Could you check a few things on this model? Use its own coordinates, in mm. A direction names the side the tool comes from. Give positions to 0.01 mm unless a question says otherwise; leave off trailing zeros. Write each loop counter-clockwise with the first axis right and the second up, starting at its lowest first coordinate (ties: lowest second). Pieces come first, ordered by that corner, then holes. Notation, with made-up numbers: (-17.75, 40.5) -> (-5.75, 40.5) arc R7 ccw to (-5.75, 51.5) -> close; hole circle Ø11 at (66, 79.25). An arc over 180 degrees is marked (long way). Write item = value, one per line. Start each with the question number.
```python
from build123d import *

# Parameters (mm, degrees)
SKETCH1_R               = 31.75
BOSS_EXTRUDE1_DEPTH     = 19.05
SKETCH2_R               = 31.75
SKETCH2_R_2             = 19.05
CUT_EXTRUDE_THIN1_DEPTH = 12.7
CUT_EXTRUDE1_DEPTH      = 49.775275499
CUT_EXTRUDE1_DEPTH_BACK = 49.775275499
SKETCH3_R               = 11
SKETCH6_R               = 11
SKETCH6_R_2             = 8.46
EXTRUDE_THIN1_DEPTH     = 12.05


with BuildPart() as part:
    # Sketch1 → Boss-Extrude1 (new, symmetric)
    with BuildSketch(Plane(origin=(0, 0, 0), x_dir=(1, 0, 0), z_dir=(0, 1, 0))):
        with Locations(Location((0, 0, 0), (0, 0, 90))):
            Circle(SKETCH1_R)
    extrude(amount=BOSS_EXTRUDE1_DEPTH, both=True)

    # Sketch2 → Cut-Extrude-Thin1 (cut, symmetric)
    with BuildSketch(Plane(origin=(0, 0, 0), x_dir=(1, 0, 0), z_dir=(0, 1, 0))):
        Circle(SKETCH2_R)
        Circle(SKETCH2_R_2, mode=Mode.SUBTRACT)
    extrude(amount=CUT_EXTRUDE_THIN1_DEPTH, both=True, mode=Mode.SUBTRACT)

    # Sketch3 → Cut-Extrude1 (cut, two sides: drawn at the far end of the back side and taken through both)
    with BuildSketch(Plane(origin=(0, 0, 0), x_dir=(1, 0, 0), z_dir=(0, 1, 0)).offset(-CUT_EXTRUDE1_DEPTH_BACK)):
        with Locations(Location((0, 0, 0), (0, 0, 270))):
            Circle(SKETCH3_R)
    extrude(amount=CUT_EXTRUDE1_DEPTH + CUT_EXTRUDE1_DEPTH_BACK, mode=Mode.SUBTRACT)

    # Sketch6 → Extrude-Thin1 (add, symmetric)
    with BuildSketch(Plane(origin=(0, 0, 0), x_dir=(1, 0, 0), z_dir=(0, 1, 0))):
        Circle(SKETCH6_R)
        Circle(SKETCH6_R_2, mode=Mode.SUBTRACT)
    extrude(amount=EXTRUDE_THIN1_DEPTH, both=True)


solid = part.part
```
(1) On a 3-axis mill with a long thin cutter (end or side, diameter ignored), from which of +Z, -Z, +X, -X, +Y, -Y can I reach the whole of each face in a straight line? I mean faces 5 (the flat face through (5.7, -12.05, 6.5)), 6 (the flat face through (14, 19.05, 0)), 7 (the flat face through (14, 12.7, 14)), 8 (the cylindrical face through (3.304, 15.501, 10.492)). Say none if no direction works.
(2) Imagine slicing it at D-D (x = 0). Please give me the cut outline in (y, z), then the cut area to 3 significant figures.
(3) I'm going to push flat-ended pins straight in: pin 1 (5 mm diameter, centred on x = 6, z = 3, fed in from -Y); pin 2 (19.5 mm diameter, centred on x = 0, z = 0, fed in from +Y); pin 3 (4 mm diameter, centred on x = 11.5, y = 3, fed in from +Z); pin 4 (24 mm diameter, centred on x = -2.5, z = -3.5, fed in from +Y). Where does each tip first touch, or does it pass through?
(4) We'd pull the mould along Y, two halves only. Please class faces 1 (the cylindrical face through (3.304, -15.599, 10.492)), 2 (the flat face through (14, -19.05, 0)), 3 (the cylindrical face through (-15.12, -0.18, 11.59)), 4 (the flat face through (14, -12.7, 14)): released by +Y, released by -Y, zero draft, split by the parting line, or undercut.
(5) Imagine slicing it at B-B (x = 26.5). Please give me the cut outline in (y, z), then the cut area to 3 significant figures.
(6) Imagine slicing it at C-C (y = 5). Please give me the cut outline in (x, z), then the cut area to 3 significant figures.
(7) Imagine slicing it at A-A (z = 0). Please give me the cut outline in (x, y), then the cut area to 3 significant figures.
(8) If I drill on line 1 along Y through (x, z) = (2.5, 22.5); line 2 along Z through (x, y) = (0, 6.5); line 3 along Z through (x, y) = (-1.5, -12), over which ranges is the centre line in solid material (lowest first)? Write a range as from..to.
Answers below:
q1.face_5 = -Y
q1.face_6 = +Z, -Z, +X, -X, +Y
q1.face_7 = none
q1.face_8 = +Y
q2.outline = (-19.05, -31.75) -> (-12.7, -31.75) -> (-12.7, -19.05) -> (12.7, -19.05) -> (12.7, -31.75) -> (19.05, -31.75) -> (19.05, -11) -> (12.05, -11) -> (12.05, -8.46) -> (-12.05, -8.46) -> (-12.05, -11) -> (-19.05, -11) -> close; (-19.05, 11) -> (-12.05, 11) -> (-12.05, 8.46) -> (12.05, 8.46) -> (12.05, 11) -> (19.05, 11) -> (19.05, 31.75) -> (12.7, 31.75) -> (12.7, 19.05) -> (-12.7, 19.05) -> (-12.7, 31.75) -> (-19.05, 31.75) -> close
q2.area = 1,060 mm^2
q3.pin_1 = -12.05
q3.pin_2 = 12.05
q3.pin_3 = 16.51
q3.pin_4 = 19.05
q4.face_1 = zero draft
q4.face_2 = released by -Y
q4.face_3 = undercut
q4.face_4 = undercut
q5.outline = (-19.05, -17.49) -> (-12.7, -17.49) -> (-12.7, 17.49) -> (-19.05, 17.49) -> close; (12.7, -17.49) -> (19.05, -17.49) -> (19.05, 17.49) -> (12.7, 17.49) -> close
q5.area = 444 mm^2
q6.outline = circle Ø38.1 at (0, 0); hole circle Ø16.92 at (0, 0)
q6.area = 915 mm^2
q7.outline = (-31.75, -19.05) -> (-11, -19.05) -> (-11, -12.05) -> (-8.46, -12.05) -> (-8.46, 12.05) -> (-11, 12.05) -> (-11, 19.05) -> (-31.75, 19.05) -> (-31.75, 12.7) -> (-19.05, 12.7) -> (-19.05, -12.7) -> (-31.75, -12.7) -> close; (8.46, -12.05) -> (11, -12.05) -> (11, -19.05) -> (31.75, -19.05) -> (31.75, -12.7) -> (19.05, -12.7) -> (19.05, 12.7) -> (31.75, 12.7) -> (31.75, 19.05) -> (11, 19.05) -> (11, 12.05) -> (8.46, 12.05) -> close
q7.area = 1,060 mm^2
q8.line_1 = -19.05..-12.7, 12.7..19.05
q8.line_2 = -19.05..-8.46, 8.46..19.05
q8.line_3 = -18.99..-8.33, 8.33..18.99
